The listing builds one solid part. Answer for the finished solid, in the listing's coordinates (mm). Give positions to 0.01 mm unless a question says otherwise; leave off trailing zeros. Loops run counter-clockwise (first coordinate to the right, second up) from the corner with the lowest first, then second, coordinate; pieces in that order, holes last. Notation, with made-up numbers: M 71.5,67.25 L 102.5,67.25 A9 ccw 102.5,83.25 Z; hole C -29,-30 d10. An arc over 180 degrees is marked long. Return JSON: item names as keys, results as strings.
from build123d import *

# Parameters (mm, degrees)
SKETCH1_W               = 185
SKETCH1_H               = 413
BASE_DEPTH              = 4
SKETCH2_W               = 20
SKETCH2_H               = 5
BOSS_EXTRUDE2_DEPTH     = 4
LPATTERN1_COUNT         = 2
LPATTERN1_PITCH         = 55
LPATTERN1_COL_COUNT     = 2
LPATTERN1_COL_PITCH     = 55
SKETCH3_W               = 4
SKETCH3_H               = 20
CUT_EXTRUDE1_DEPTH      = 231.877673238
LPATTERN2_COUNT         = 4
LPATTERN2_PITCH         = 55
LPATTERN2_COL_COUNT     = 4
LPATTERN2_COL_PITCH     = 55
FILLET1_R               = 10
MIRROR1_COPY_1_SKETCH_W = 20
MIRROR1_COPY_1_SKETCH_H = 5
MIRROR1_COPY_1_DEPTH    = 4
MIRROR1_COPY_2_SKETCH_W = 20
MIRROR1_COPY_2_SKETCH_H = 5
MIRROR1_COPY_2_DEPTH    = 4
CUT_EXTRUDE4_DEPTH      = 231.877673238
LPATTERN5_COUNT         = 4
LPATTERN5_PITCH         = 117.666666667


with BuildPart() as part:
    # Sketch1 → Base (new body)
    with BuildSketch(Plane(origin=(0, 0, 0), x_dir=(1, 0, 0), z_dir=(0, 1, 0))):
        Rectangle(SKETCH1_W, SKETCH1_H)
    extrude(amount=BASE_DEPTH)

    # Sketch2 → Boss-Extrude2 (add)
    with BuildSketch(Plane(origin=(0, 4, 0), x_dir=(1, 0, 0), z_dir=(0, 1, 0))):
        with Locations((0, -209)):
            Rectangle(SKETCH2_W, SKETCH2_H)
    boss_extrude2 = extrude(amount=-BOSS_EXTRUDE2_DEPTH)

    # LPattern1: Boss-Extrude2 ×2
    with Locations(*[(-i * LPATTERN1_PITCH, 0, 0) for i in range(1, LPATTERN1_COUNT)]):
        add(boss_extrude2)

    # LPattern1 col: Boss-Extrude2 ×2
    with Locations(*[(i * LPATTERN1_COL_PITCH, 0, 0) for i in range(1, LPATTERN1_COL_COUNT)]):
        add(boss_extrude2)

    # Sketch3 → Cut-Extrude1 (cut, through all)
    with BuildSketch(Plane(origin=(0, 4, 0), x_dir=(1, 0, 0), z_dir=(0, 1, 0))):
        with Locations((-85.5, 0)):
            Rectangle(SKETCH3_W, SKETCH3_H)
    cut_extrude1 = extrude(amount=-CUT_EXTRUDE1_DEPTH, mode=Mode.SUBTRACT)

    # LPattern2: Cut-Extrude1 ×4
    with Locations(*[(0, 0, -i * LPATTERN2_PITCH) for i in range(1, LPATTERN2_COUNT)]):
        add(cut_extrude1, mode=Mode.SUBTRACT)

    # LPattern2 col: Cut-Extrude1 ×4
    with Locations(*[(0, 0, i * LPATTERN2_COL_PITCH) for i in range(1, LPATTERN2_COL_COUNT)]):
        add(cut_extrude1, mode=Mode.SUBTRACT)

    # Fillet1
    fillet1_edges = [part.edges().sort_by_distance(p)[0] for p in [
        (-92.5, 2, -206.5),
        (92.5, 2, -206.5),
        (92.5, 2, 206.5),
        (-92.5, 2, 206.5),
    ]]
    fillet(fillet1_edges, radius=FILLET1_R)

    # Mirror1: Boss-Extrude2 across plane
    add(boss_extrude2.mirror(Plane.XY))

    # Mirror1 copy 1 sketch → Mirror1 copy 1 (add)
    with BuildSketch(Plane(origin=(-55, 4, 0), x_dir=(1, 0, 0), z_dir=(0, 1, 0))):
        with Locations((0, 209)):
            Rectangle(MIRROR1_COPY_1_SKETCH_W, MIRROR1_COPY_1_SKETCH_H)
    extrude(amount=-MIRROR1_COPY_1_DEPTH)

    # Mirror1 copy 2 sketch → Mirror1 copy 2 (add)
    with BuildSketch(Plane(origin=(55, 4, 0), x_dir=(1, 0, 0), z_dir=(0, 1, 0))):
        with Locations((0, 209)):
            Rectangle(MIRROR1_COPY_2_SKETCH_W, MIRROR1_COPY_2_SKETCH_H)
    extrude(amount=-MIRROR1_COPY_2_DEPTH)

    # Sketch5 → Cut-Extrude4 (cut, through all)
    with BuildSketch(Plane(origin=(0, 4, 0), x_dir=(1, 0, 0), z_dir=(0, 1, 0))):
        Polygon((-46.895000001, 87.351848615), (-61.230000001, 87.351848615), (-61.230000001, 102.480848615), (-68.500000001, 102.480848615), (-68.500000001, 45.870848615), (-61.230000001, 45.870848615), (-61.230000001, 50.331848615), (-49.211989258, 50.331848615), (-49.211989258, 67.349848615), (-46.895000001, 67.349848615), align=None)
        Polygon((-46.895000001, 147.351848615), (-61.230000001, 147.351848615), (-61.230000001, 162.480848615), (-68.500000001, 162.480848615), (-68.500000001, 105.870848615), (-61.230000001, 105.870848615), (-61.230000001, 110.331848615), (-49.211989258, 110.331848615), (-49.211989258, 127.349848615), (-46.895000001, 127.349848615), align=None)
    extrude(amount=-CUT_EXTRUDE4_DEPTH, mode=Mode.SUBTRACT)

    # Sketch8 → Tap Drill for M2.5x0.45 Tap1 (revolve, cut)
    with BuildSketch(Plane(origin=(92.5, 2, -176.5), x_dir=(0, 0, -1), z_dir=(0, 1, 0))):
        Polygon((0, 0), (0, 5.615882135), (1.025, 5), (1.025, 0), align=None)
    tap_drill_for_m2_5x0_45_tap1 = revolve(axis=Axis((98.85, 2, -176.5), (-1, 0, 0)), mode=Mode.SUBTRACT)

    # LPattern5: Tap Drill for M2.5x0.45 Tap1 ×4
    with Locations(*[(0, 0, i * LPATTERN5_PITCH) for i in range(1, LPATTERN5_COUNT)]):
        add(tap_drill_for_m2_5x0_45_tap1, mode=Mode.SUBTRACT)


solid = part.part
(1) Given pin 1 (1.2 mm diameter, centred on x = -84.5, y = 1.5, fed in from -Z); pin 2 (1.2 mm diameter, centred on y = 1.5, z = 208.5, fed in from -X), each flat-ended and moving along its own axis, determine where each tip first touches the part or whether it passes through.
Values follow:
{"pin 1": "z = -206.4", "pin 2": "x = -65"}
(2) The part is cut by section A-A (x = -18). Determine the outline of the cut face in (y, z), and give its area (3 significant figures).
Values follow:
{"outline": "M 0,-206.5 L 4,-206.5 L 4,206.5 L 0,206.5 Z", "area": "1,650 mm²"}
(3) Straight lines are drawn through the part: line 1 along X through (y, z) = (2.9, -162); line 2 along X through (y, z) = (3.45, -115); line 3 along Z through (x, y) = (-54, 0.4). For each, find the intervals that lie inside material, in ascending order.
Values follow:
{"line 1": "-92.5 to -87.5, -83.5 to -68.5, -61.23 to 92.5", "line 2": "-92.5 to -87.5, -83.5 to -68.5, -49.21 to 92.5", "line 3": "-211.5 to -147.35, -110.33 to -87.35, -50.33 to 211.5"}
